Source: CAD feature listing. Evaluate the final solid. Frame: model axes, mm. A direction names the side the tool comes from. Give positions to 0.01 mm unless a question says otherwise; leave off trailing zeros. Order: outer loops, then holes, each group sorted by start corner. A loop starts at its lowest first (then second) coordinate and runs counter-clockwise, first axis right, second up. Notation, with made-up numbers: M -8.75,53.5 L 8.25,53.5 A20 cw 8.25,86.5 Z; hole C -23.5,57 d9. An arc over 180 degrees is marked long. Return JSON: item names as keys, results as strings.
from build123d import *

# Parameters (mm, degrees)
F0_R     = 6.975
F0_R_2   = 5.625
F0_R_3   = 1
F0_R_4   = 0.75
F1_DEPTH = 3
F2_SIZE2 = 1.8
F2_SIZE  = 2.8
F4_DEPTH = 2.3
F5_DEPTH = 1.6


with BuildPart() as f1:
    # F0 (on Top) → F1 (new body)
    with BuildSketch(Plane.XY):
        Circle(F0_R)
        Circle(F0_R_2, mode=Mode.SUBTRACT)
        Circle(F0_R_2)
        with Locations((0, -2.5)):
            Circle(F0_R_3, mode=Mode.SUBTRACT)
        with Locations((-2.5, 0)):
            Circle(F0_R_3, mode=Mode.SUBTRACT)
        Circle(F0_R_4, mode=Mode.SUBTRACT)
        with Locations((2.5, 0)):
            Circle(F0_R_3, mode=Mode.SUBTRACT)
        with Locations((0, 2.5)):
            Circle(F0_R_3, mode=Mode.SUBTRACT)
    extrude(amount=F1_DEPTH)

    # F2
    f2_edges = [f1.edges().sort_by_distance(p)[0] for p in [
        (-6.975, 0, 3),
    ]]
    f2_side = f1.faces().sort_by_distance((-6.777717, 0, 3))[0]
    chamfer(f2_edges, length=F2_SIZE, length2=F2_SIZE2, reference=f2_side)

    # F3 (on face) → F4 (cut, through all)
    with BuildSketch(Plane.XY.offset(3)):
        with BuildLine():
            Line((-1.475, 4.8497422612), (-1.475, 6.8172575131))
            ThreePointArc((-1.475, 6.8172575131), (-3.4875, 6.0405271914), (-5.1664181905, 4.6860162271))
            Line((-5.1664181905, 4.6860162271), (-3.4625, 3.7022586012))
            ThreePointArc((-3.4625, 3.7022586012), (-2.1375, 3.7022586012), (-1.475, 4.8497422612))
        make_face()
        with BuildLine():
            Line((1.475, 6.8172575131), (1.475, 4.8497422612))
            ThreePointArc((1.475, 4.8497422612), (2.1375, 3.7022586012), (3.4625, 3.7022586012))
            Line((3.4625, 3.7022586012), (5.1664181905, 4.6860162271))
            ThreePointArc((5.1664181905, 4.6860162271), (3.4875, 6.0405271914), (1.475, 6.8172575131))
        make_face()
        with BuildLine():
            Line((6.6414181905, 2.131241286), (4.9375, 1.14748366))
            ThreePointArc((4.9375, 1.14748366), (4.275, 0), (4.9375, -1.14748366))
            Line((4.9375, -1.14748366), (6.6414181905, -2.131241286))
            ThreePointArc((6.6414181905, -2.131241286), (6.975, 0), (6.6414181905, 2.131241286))
        make_face()
        with BuildLine():
            Line((5.1664181905, -4.6860162271), (3.4625, -3.7022586012))
            ThreePointArc((3.4625, -3.7022586012), (2.1375, -3.7022586012), (1.475, -4.8497422612))
            Line((1.475, -4.8497422612), (1.475, -6.8172575131))
            ThreePointArc((1.475, -6.8172575131), (3.4875, -6.0405271914), (5.1664181905, -4.6860162271))
        make_face()
        with BuildLine():
            ThreePointArc((-1.475, -4.8497422612), (-2.1375, -3.7022586012), (-3.4625, -3.7022586012))
            Line((-3.4625, -3.7022586012), (-5.1664181905, -4.6860162271))
            ThreePointArc((-5.1664181905, -4.6860162271), (-3.4875, -6.0405271914), (-1.475, -6.8172575131))
            Line((-1.475, -6.8172575131), (-1.475, -4.8497422612))
        make_face()
        with BuildLine():
            ThreePointArc((-4.9375, -1.14748366), (-4.275, 0), (-4.9375, 1.14748366))
            Line((-4.9375, 1.14748366), (-6.6414181905, 2.131241286))
            ThreePointArc((-6.6414181905, 2.131241286), (-6.975, 0), (-6.6414181905, -2.131241286))
            Line((-6.6414181905, -2.131241286), (-4.9375, -1.14748366))
        make_face()
    extrude(amount=-F4_DEPTH, mode=Mode.SUBTRACT)

    # F0 (on Top) → F5 (cut, through all)
    with BuildSketch(Plane.XY):
        Circle(F0_R_2)
        with Locations((0, -2.5)):
            Circle(F0_R_3, mode=Mode.SUBTRACT)
        with Locations((-2.5, 0)):
            Circle(F0_R_3, mode=Mode.SUBTRACT)
        Circle(F0_R_4, mode=Mode.SUBTRACT)
        with Locations((2.5, 0)):
            Circle(F0_R_3, mode=Mode.SUBTRACT)
        with Locations((0, 2.5)):
            Circle(F0_R_3, mode=Mode.SUBTRACT)
    extrude(amount=F5_DEPTH, mode=Mode.SUBTRACT)


solid = f1.part
1. Set-up query: faces 4 (the face through (-1, 0, 1.6)), 5 (the face through (6, 0, 0.7)), 6 (the face through (-5.801, -1.646, 1.383)), 7 (the face through (-5, 3, 0)), 8 (the face through (-4.326, 4.201, 1.383)). Return all of +Z, -Z, +X, -X, +Y, -Y with unobstructed straight access to the full face (end or side cutting, diameter ignored); none if empty.
Evaluation:
{"face 4": "-Z", "face 5": "+Z, +X", "face 6": "+Z, -X", "face 7": "-Z, +X, -X, +Y, -Y", "face 8": "+Z, +Y"}
2. Section query A-A (y = 0). Return loops of the section in (x, z) (3 decimals).
Evaluation:
{"outline": "M -6.975,0 L -5.625,0 L -5.625,0.7 L -6.975,0.7 Z; M -4.275,1.6 L -3.5,1.6 L -3.5,3 L -4.175,3 L -4.275,2.936 Z; M -1.5,1.6 L -0.75,1.6 L -0.75,3 L -1.5,3 Z; M 0.75,1.6 L 1.5,1.6 L 1.5,3 L 0.75,3 Z; M 3.5,1.6 L 4.275,1.6 L 4.275,2.936 L 4.175,3 L 3.5,3 Z; M 5.625,0 L 6.975,0 L 6.975,0.7 L 5.625,0.7 Z"}
3. Ray query, probe 1 along Y at (x, z) = (0, 0.75) (3 decimals); probe 2 along Y at (x, z) = (0, 2.7); probe 3 along X at (y, z) = (0.25, 1.9). Return the intervals inside material, ascending.
Evaluation:
{"probe 1": "y = -6.975 to -5.625, 5.625 to 6.975", "probe 2": "y = -4.64 to -3.5, -1.5 to -0.75, 0.75 to 1.5, 3.5 to 4.64", "probe 3": "x = -4.3 to -3.47, -1.53 to -0.71, 0.71 to 1.53, 3.47 to 4.3"}
4. Section query C-C (x = -2.75). State how many separate pieces and enclosed holes the cut face has, then the cut area to 3 significant figures.
Evaluation:
{"separate pieces": "4", "enclosed holes": "0", "area": "9.19 mm^2"}
5. Section query B-B (x = 0). Return loops of the section in (y, z) (3 decimals), then the cut area to 3 significant figures.
Evaluation:
{"outline": "M -6.975,0 L -5.625,0 L -5.625,1.6 L -3.5,1.6 L -3.5,3 L -4.175,3 L -6.975,1.2 Z; M -1.5,1.6 L -0.75,1.6 L -0.75,3 L -1.5,3 Z; M 0.75,1.6 L 1.5,1.6 L 1.5,3 L 0.75,3 Z; M 3.5,1.6 L 5.625,1.6 L 5.625,0 L 6.975,0 L 6.975,1.2 L 4.175,3 L 3.5,3 Z", "area": "11.1 mm^2"}
6. First-contact query: pin 1 (1.4 mm diameter, centred on y = 5.5, z = 1.5, fed in from -X); pin 2 (2.5 mm diameter, centred on x = -3.5, y = -5.5, fed in from +Z); pin 3 (1 mm diameter, centred on y = 0, z = 2, fed in from +X); pin 4 (1.6 mm diameter, centred on x = 0, y = -2.5, fed in from +Z). Flat tips, straight axial feed; report the tip coordinate or a pass-through.
Evaluation:
{"pin 1": "stops at x = -1.48", "pin 2": "stops at z = 0.7", "pin 3": "stops at x = 4.37", "pin 4": "passes through"}
7. Draft query along Y for faces 1 (the face through (-6, 0, 0.7)), 2 (the face through (-3, 5, 0.7)), 3 (the face through (4.326, -4.201, 1.383)). Return one class per face: pulls with the +Y half, pulls with the -Y half, needs draft (parallel to the pull), parting line crosses it, or undercut.
Evaluation:
{"face 1": "undercut", "face 2": "needs draft", "face 3": "pulls with the -Y half"}
